Part print with two shaded views. Sizes in mm from the minimum x, y, z corner. A direction names the side the tool comes from. Coordinates: 2 decimals unless noted, no trailing zeros. Write each loop counter-clockwise with the first axis right and the second up, starting at its lowest first coordinate (ties: lowest second). Pieces come first, ordered by that corner, then holes. Notation, with made-up numbers: (13.25, -17.75) - (22.25, -17.75) arc R24 ccw to (22.25, -1.75) - close; hole circle Ø6 at (23, 64.25). An arc over 180 degrees is marked (long way). Answer in a Markdown table with one row per item. Add a question column.
Q1. Band-saw the part on C-C (y = 19). List the corners of the cut face in (x, z) (3 decimals), and give its area (4 significant figures).
Q2. Pin check, flat tips, straight feed: pin 1 (5 mm diameter, centred on y = 5.5, z = 15.5, fed in from -X); pin 2 (2 mm diameter, centred on x = 25, z = 21, fed in from -Y); pin 3 (0.8 mm diameter, centred on x = 48.5, z = 21.5, fed in from +Y); pin 4 (5 mm diameter, centred on x = 21.5, z = 14.5, fed in from +Y). Stop position of each tip, or through.
Q3. Band-saw the part on B-B (z = 19). List the corners of the cut face in (x, y).
Q4. 3-axis set-ups, long thin cutter, end or side, ignore diameter. For the marked faces 1, 2 and 3: which of +Z, -Z, +X, -X, +Y, -Y reach the whole face in a straight line?
Q5. Band-saw the part on A-A (x = 31.5). List the corners of the cut face in (y, z), and give its area (3 significant figures).
Q6. Band-saw the part on D-D (x = 7.5). List the corners of the cut face in (y, z).
Q7. Drill centre lines: line 1 along X through (y, z) = (14.75, 29); line 2 along Y through (x, z) = (14, 22.5); line 3 along Z through (x, y) = (34.5, 18). Where is each one in solid material? Low to high. Write a range as from..to.
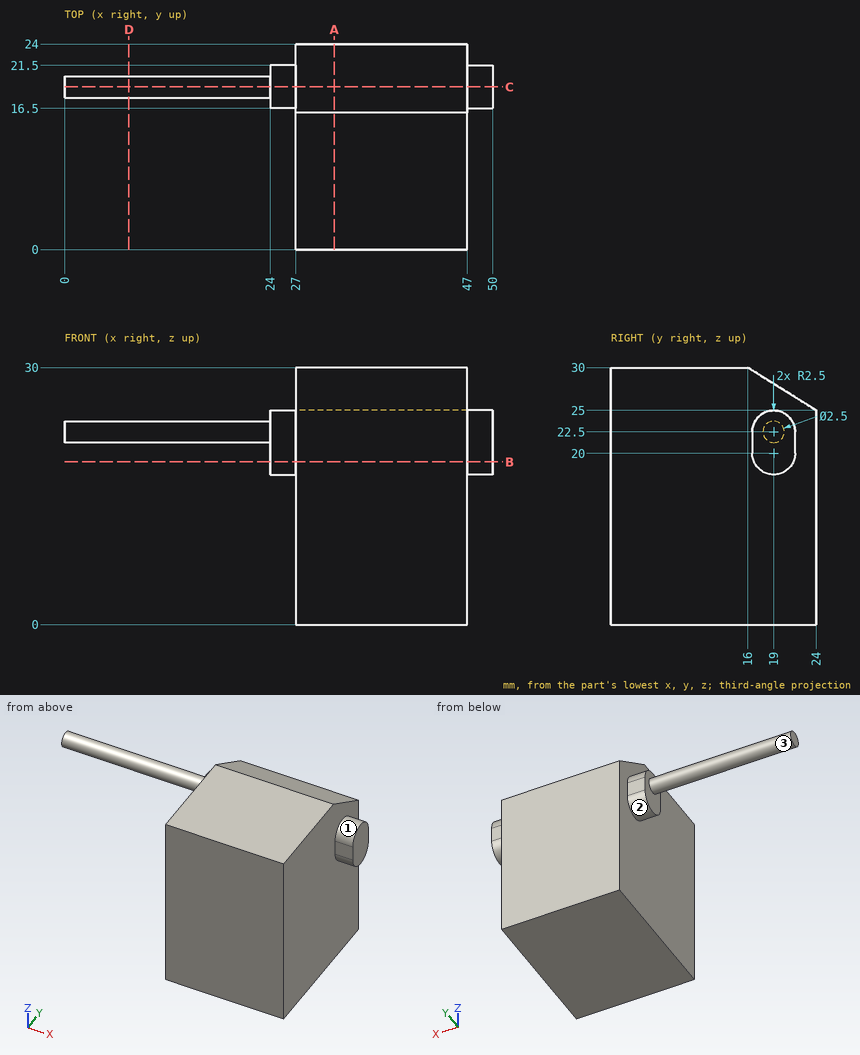
Checked values:
| question | item | result |
|---|---|---|
| 1 | outline | (0, 21.25) - (24, 21.25) - (24, 17.5) - (27, 17.5) - (27, 0) - (47, 0) - (47, 17.5) - (50, 17.5) - (50, 25) - (47, 25) - (47, 28.125) - (27, 28.125) - (27, 25) - (24, 25) - (24, 23.75) - (0, 23.75) - close |
| 1 | area | 667.5 mm² |
| 2 | pin 1 | stops at x = 27 |
| 2 | pin 2 | stops at y = 16.5 |
| 2 | pin 3 | stops at y = 21.5 |
| 2 | pin 4 | passes through |
| 3 | outline | (24, 16.71) - (27, 16.71) - (27, 0) - (47, 0) - (47, 16.71) - (50, 16.71) - (50, 21.29) - (47, 21.29) - (47, 24) - (27, 24) - (27, 21.29) - (24, 21.29) - close |
| 4 | face 1 | +Z, +X |
| 4 | face 2 | -Z, -X |
| 4 | face 3 | -X |
| 5 | outline | (0, 0) - (24, 0) - (24, 25) - (16, 30) - (0, 30) - close |
| 5 | area | 700 mm² |
| 6 | outline | circle Ø2.5 at (19, 22.5) |
| 7 | line 1 | x = 27..47 |
| 7 | line 2 | y = 17.75..20.25 |
| 7 | line 3 | z = 0..28.75 |
